CAD build for the part. Positions are in the model's coordinates, mm. Face numbers are marked on the shaded views. A direction names the side the tool comes from. Coordinates: 2 decimals unless noted, no trailing zeros. Loops run counter-clockwise (first coordinate to the right, second up) from the corner with the lowest first, then second, coordinate; pieces in that order, holes last.
1) Saw through at C-C, the plane z = 15. Write the cut outline in (x, y).
2) Wall check: line 1 along Y through (x, z) = (-7, -0.5); line 2 along Y through (x, z) = (-22, -1.5); line 3 along Y through (x, z) = (-22, 2). Give the ranges that are in metal, low to high.
3) Which spindle directions (+Z, -Z, +X, -X, +Y, -Y) get a long thin tool onto all of the face, cutting with end or side? Do the marked faces 1, 2, 3, 4 and 5. Say none if no direction does.
4) Saw through at A-A, the plane y = 0. Write the cut outline in (x, z), and give its area (3 significant figures).
5) Pin check, flat tips, straight feed: pin 1 Ø0.6 at (x, y) = (-31, 4.5) entering from +Z; pin 2 Ø1.5 at (x, z) = (-5, -1.5) entering from -Y; pin 3 Ø3 at (x, z) = (-30, -1) entering from +Y. Stop position of each tip, or through.
6) Saw through at D-D, the plane x = 6. Write the cut outline in (y, z).
7) Saw through at B-B, the plane z = -1. Write the cut outline in (x, y), and give its area (3 significant figures).
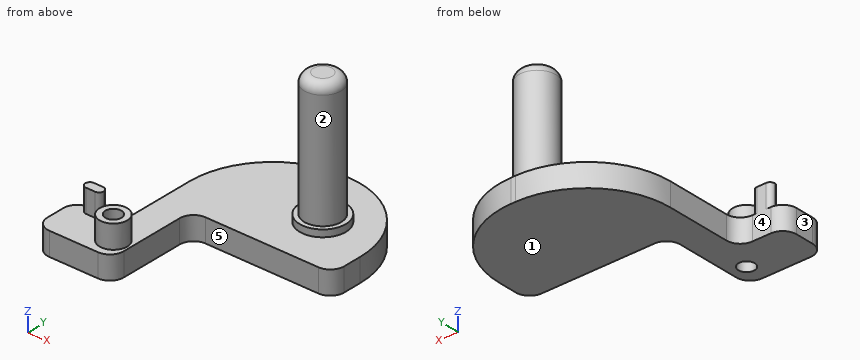
```python
from build123d import *

# Parameters (mm, degrees)
F0_R      = 5
F0_R_2    = 1.75
F0_W      = 10
F0_H      = 10
F0_R_3    = 4
F1_DEPTH  = 5
F2_DEPTH  = 1.5
F3_R      = 4
F4_DEPTH  = 27
F5_R      = 2
F6_R      = 18
F7_R      = 3
F7_R_2    = 1.75
F8_DEPTH  = 5
F9_R      = 3
F10_W     = 4
F10_H     = 2
F11_DEPTH = 5
F12_R     = 0.99999


# Not quite as in the source:
# - a fillet or chamfer is up to 0.001 mm smaller than in the source, because OpenCascade refuses the exact size


with BuildPart() as f1:
    # F0 (on Top) → F1 (new body)
    with BuildSketch(Plane.XY):
        Polygon((-25, 15.5), (-18.459414942, 15.5), (12, 15.5), (12, 40.5), (-25, 40.5), align=None)
        with Locations((0, 27)):
            Circle(F0_R, mode=Mode.SUBTRACT)
        Polygon((-25, 5.5), (-25, -4.5), (-18.459414942, -4.5), (-18.459414942, 15.5), (-25, 15.5), align=None)
        with Locations((-22, 0)):
            Circle(F0_R_2, mode=Mode.SUBTRACT)
        with Locations((-30, 0.5)):
            Rectangle(F0_W, F0_H)
        with Locations((0, 27)):
            Circle(F0_R)
        with Locations((0, 27)):
            Circle(F0_R_3, mode=Mode.SUBTRACT)
        with Locations((0, 27)):
            Circle(F0_R_3)
    extrude(amount=-F1_DEPTH)

    # F0 (on Top) → F2 (join)
    with BuildSketch(Plane.XY):
        with Locations((0, 27)):
            Circle(F0_R)
        with Locations((0, 27)):
            Circle(F0_R_3, mode=Mode.SUBTRACT)
        with Locations((0, 27)):
            Circle(F0_R_3)
    extrude(amount=F2_DEPTH)

    # F3 (on face) → F4 (join)
    with BuildSketch(Plane.XY.offset(1.5)):
        with Locations((0, 27)):
            Circle(F3_R)
    extrude(amount=F4_DEPTH)

    # F5
    f5_edges = [f1.edges().sort_by_distance(p)[0] for p in [
        (-4, 27, 28.5),
    ]]
    fillet(f5_edges, radius=F5_R)

    # F6
    f6_edges = [f1.edges().sort_by_distance(p)[0] for p in [
        (-25, 40.5, -2.5),
        (12, 40.5, -2.5),
    ]]
    fillet(f6_edges, radius=F6_R)

    # F7 (on face) → F8 (join)
    with BuildSketch(Plane.XY):
        with Locations((-22, 0)):
            Circle(F7_R)
        with Locations((-22, 0)):
            Circle(F7_R_2, mode=Mode.SUBTRACT)
    extrude(amount=F8_DEPTH)

    # F9
    f9_edges = [f1.edges().sort_by_distance(p)[0] for p in [
        (-25, 5.5, -2.5),
        (-35, 5.5, -2.5),
        (-35, -4.5, -2.5),
        (-18.459415, -4.5, -2.5),
        (-18.459415, 15.5, -2.5),
        (12, 15.5, -2.5),
    ]]
    fillet(f9_edges, radius=F9_R)

    # F10 (on face) → F11 (join)
    with BuildSketch(Plane.XY):
        with Locations((-30, 4.5)):
            Rectangle(F10_W, F10_H)
    extrude(amount=F11_DEPTH)

    # F12 (radius 1 in the source; OpenCascade refuses exactly that, so slightly less here)
    f12_edges = [f1.edges().sort_by_distance(p)[0] for p in [
        (-32, 5.5, 2.5),
        (-32, 3.5, 2.5),
        (-28, 3.5, 2.5),
        (-28, 5.5, 2.5),
    ]]
    fillet(f12_edges, radius=F12_R)


solid = f1.part
```
Data:
1. outline: circle Ø8 at (0, 27)
2. line 1: y = 15.5 to 40.5
2. line 2: y = -4.5 to -1.75, 1.75 to 32.45
2. line 3: y = -3 to -1.75, 1.75 to 3
3. face 1: -Z, +X, -X, +Y, -Y
3. face 2: +Z
3. face 3: +Z, -Z, -X, +Y, -Y
3. face 4: +Z, -Z, -X, +Y
3. face 5: +Z, -Z, +X, -Y
4. outline: (-35, -5) - (-23.75, -5) - (-23.75, 5) - (-25, 5) - (-25, 0) - (-35, 0) - close; (-20.25, -5) - (-18.46, -5) - (-18.46, 0) - (-19, 0) - (-19, 5) - (-20.25, 5) - close
4. area: 77.7 mm2
5. pin 1: stops at z = 5
5. pin 2: stops at y = 15.5
5. pin 3: stops at y = 5.5
6. outline: (15.5, -5) - (35.92, -5) - (35.92, 0) - (15.5, 0) - close
7. outline: (-35, -1.5) arc R3 ccw to (-32, -4.5) - (-21.46, -4.5) arc R3 ccw to (-18.46, -1.5) - (-18.46, 12.5) arc R3 cw to (-15.46, 15.5) - (9, 15.5) arc R3 ccw to (12, 18.5) - (12, 22.5) arc R18 ccw to (-6, 40.5) - (-7, 40.5) arc R18 ccw to (-25, 22.5) - (-25, 8.5) arc R3 cw to (-28, 5.5) - (-32, 5.5) arc R3 ccw to (-35, 2.5) - close; hole circle Ø3.5 at (-22, 0)
7. area: 1,000 mm2
